from build123d import *

# Parameters (mm, degrees)
F1_DEPTH = 58.75
F0_R     = 2.35
F2_DEPTH = 1
F3_W     = 28.5
F3_H     = 38.25
F4_DEPTH = 9.75
F5_W     = 43
F5_H     = 37.5
F6_DEPTH = 10.5
F7_W     = 4.8
F7_H     = 0.5
F8_DEPTH = 8.75
F9_SIZE  = 0.75


with BuildPart() as f1:
    # F0 (on Top) → F1 (new body)
    with BuildSketch(Plane.XY):
        Polygon((11.05, -24.925), (14.325, -24.925), (14.325, 24.925), (11.05, 24.925), (-11.05, 24.925), (-14.325, 24.925), (-14.325, -24.925), (-11.05, -24.925), align=None)
    extrude(amount=F1_DEPTH)

    # F0 (on Top) → F2 (join)
    with BuildSketch(Plane.XY):
        with BuildLine():
            ThreePointArc((-11.05, -24.925), (0, -35.975), (11.05, -24.925))
            Line((11.05, -24.925), (-11.05, -24.925))
        make_face()
        with Locations((0, -30.525)):
            Circle(F0_R, mode=Mode.SUBTRACT)
        with BuildLine():
            Line((-11.05, 24.925), (11.05, 24.925))
            ThreePointArc((11.05, 24.925), (0, 35.975), (-11.05, 24.925))
        make_face()
        with Locations((0, 30.525)):
            Circle(F0_R, mode=Mode.SUBTRACT)
    extrude(amount=F2_DEPTH)

    # F3 (on face) → F4 (join)
    with BuildSketch(Plane(origin=(-14.325, 0, 0), x_dir=(0, -1, 0), z_dir=(-1, 0, 0))):
        with Locations((0, 28.875)):
            Rectangle(F3_W, F3_H)
    extrude(amount=F4_DEPTH)

    # F5 (on face) → F6 (join)
    with BuildSketch(Plane.YZ.offset(14.325)):
        with Locations((0, 29.5)):
            Rectangle(F5_W, F5_H)
    extrude(amount=F6_DEPTH)

    # F7 (on face) → F8 (join)
    with BuildSketch(Plane.YZ.offset(24.825)):
        with Locations((-18.75, 29.5)):
            Rectangle(F7_W, F7_H)
        with Locations((-18.75, 35.7)):
            Rectangle(F7_W, F7_H)
        with Locations((-18.75, 41.9)):
            Rectangle(F7_W, F7_H)
        with Locations((-18.75, 17.1)):
            Rectangle(F7_W, F7_H)
        with Locations((-18.75, 23.3)):
            Rectangle(F7_W, F7_H)
        with Locations((18.75, 29.5)):
            Rectangle(F7_W, F7_H)
        with Locations((18.75, 35.7)):
            Rectangle(F7_W, F7_H)
        with Locations((18.75, 17.1)):
            Rectangle(F7_W, F7_H)
        with Locations((18.75, 23.3)):
            Rectangle(F7_W, F7_H)
        with Locations((18.75, 41.9)):
            Rectangle(F7_W, F7_H)
    extrude(amount=F8_DEPTH)

    # F9
    f9_edges = [f1.edges().sort_by_distance(p)[0] for p in [
        (33.575, -21.15, 41.9),
        (33.575, -16.35, 41.9),
        (33.575, -21.15, 35.7),
        (33.575, -16.35, 35.7),
        (33.575, -21.15, 29.5),
        (33.575, -16.35, 29.5),
        (33.575, -21.15, 17.1),
        (33.575, -16.35, 17.1),
        (33.575, 16.35, 17.1),
        (33.575, 21.15, 17.1),
        (33.575, 16.35, 29.5),
        (33.575, 21.15, 29.5),
        (33.575, 16.35, 35.7),
        (33.575, 21.15, 35.7),
        (33.575, 16.35, 41.9),
        (33.575, 21.15, 41.9),
        (33.575, -16.35, 23.3),
        (33.575, -21.15, 23.3),
        (33.575, 16.35, 23.3),
        (33.575, 21.15, 23.3),
    ]]
    chamfer(f9_edges, length=F9_SIZE)


solid = f1.part
For this review, take the finished solid that the model builds, in its own axes (mm). A direction names the side the tool comes from. Round coordinates to 2 decimals unless told otherwise and drop trailing zeros. Write each loop counter-clockwise with the first axis right and the second up, starting at its lowest first coordinate (ties: lowest second). Pieces come first, ordered by that corner, then holes. Notation, with made-up numbers: (-24, 30) - (-20, 30) arc R16 cw to (-20, 53) - close; hole circle Ø11 at (66.25, 34.5). An arc over 180 degrees is marked (long way). Write item = value, one per line. Start each with the question number.
1. Consider section C-C on z = 45. State the section outline as (x, y) points (3 decimals).
2. Draft analysis for pull direction X (two halves, no side actions). For faces 1 (the face through (-0.51, -32.82, 0.49)), 2 (the face through (29, 19, 42.15)), 3 (the face through (-24.075, 0, 29)), 4 (the face through (-0.51, 28.23, 0.49)), state which applies: released by +X, released by -X, zero draft, split by the parting line, or undercut.
3. Wall thickness on L1, parallel to Y at x = 0, z = 0.5 (3 decimals); L2, parallel to X at y = -16, z = 21.5 (3 decimals); L3, parallel to X at y = -9, z = 18 (3 decimals): over which ranges is each line inside the solid? List them lowest first.
4. For pin 1 Ø5.5 at (x, y) = (28.5, -18) entering from +Z; pin 2 Ø1.4 at (x, y) = (28, 17.5) entering from -Z; pin 3 Ø8 at (x, y) = (27.5, -20) entering from -Z, all flat-tipped, find the tip position at first contact; note any pin that passes through.
5. Consider section B-B on y = -11. State the section outline as (x, z) points (3 decimals), plus the area to 3 significant figures.
6. Consider section D-D on x = 19. State the section outline as (y, z) points.
7. For faces 5 (the face through (-19, -14.25, 29)), 6 (the face through (29, 19, 29.75)), 7 (the face through (-19, 0, 9.75)), 8 (the face through (-19, 0, 48)), list the 3-axis set-ups (+Z, -Z, +X, -X, +Y, -Y) from which the entire face can be reached by the end or side of a thin tool; tool diameter is ignored.
8. Consider section A-A on x = 0. State the section outline as (y, z) points (3 decimals), plus the area to 3 significant figures.
Evaluation:
q1.outline = (-24.075, -14.25) - (-14.325, -14.25) - (-14.325, -24.925) - (14.325, -24.925) - (14.325, -21.5) - (24.825, -21.5) - (24.825, 21.5) - (14.325, 21.5) - (14.325, 24.925) - (-14.325, 24.925) - (-14.325, 14.25) - (-24.075, 14.25) - close
q2.face_1 = undercut
q2.face_2 = zero draft
q2.face_3 = released by -X
q2.face_4 = undercut
q3.L1 = -35.975 to -32.875, -28.175 to 28.175, 32.875 to 35.975
q3.L2 = -14.325 to 24.825
q3.L3 = -24.075 to 24.825
q4.pin_1 = 42.15
q4.pin_2 = 16.85
q4.pin_3 = 10.75
q5.outline = (-24.075, 9.75) - (-14.325, 9.75) - (-14.325, 0) - (14.325, 0) - (14.325, 10.75) - (24.825, 10.75) - (24.825, 48.25) - (14.325, 48.25) - (14.325, 58.75) - (-14.325, 58.75) - (-14.325, 48) - (-24.075, 48) - close
q5.area = 2,450 mm2
q6.outline = (-21.5, 10.75) - (21.5, 10.75) - (21.5, 48.25) - (-21.5, 48.25) - close
q7.face_5 = +Z, -Z, -X, -Y
q7.face_6 = +X, +Y, -Y
q7.face_7 = -Z, -X, +Y, -Y
q7.face_8 = +Z, -X, +Y, -Y
q8.outline = (-35.975, 0) - (-32.875, 0) - (-32.875, 1) - (-35.975, 1) - close; (-28.175, 0) - (28.175, 0) - (28.175, 1) - (24.925, 1) - (24.925, 58.75) - (-24.925, 58.75) - (-24.925, 1) - (-28.175, 1) - close; (32.875, 0) - (35.975, 0) - (35.975, 1) - (32.875, 1) - close
q8.area = 2,940 mm2
